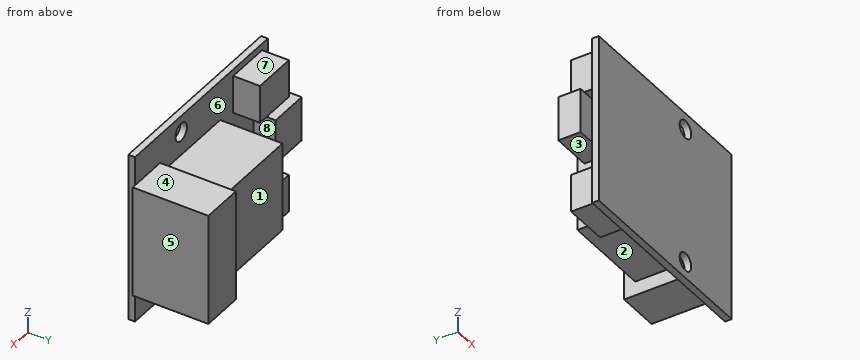
```python
from build123d import *

# Parameters (mm, degrees)
ESBO_O1_W                = 46
ESBO_O1_H                = 38
ESBO_O1_R                = 2
RESSALTO_EXTRUS_O1_DEPTH = 1.5
ESBO_O2_W                = 9
ESBO_O2_H                = 10
RESSALTO_EXTRUS_O2_DEPTH = 5
ESBO_O2_3_W              = 10
ESBO_O2_3_H              = 8.5
RESSALTO_EXTRUS_O3_DEPTH = 6
ESBO_O2_4_W              = 20
ESBO_O2_4_H              = 20
RESSALTO_EXTRUS_O4_DEPTH = 14
ESBO_O2_5_W              = 9.5
ESBO_O2_5_H              = 25
RESSALTO_EXTRUS_O5_DEPTH = 17


with BuildPart() as part:
    # Esboço1 → Ressalto-extrusão1 (new body)
    with BuildSketch(Plane(origin=(0, 0, 0), x_dir=(1, 0, 0), z_dir=(0, 1, 0))):
        Rectangle(ESBO_O1_W, ESBO_O1_H)
        with Locations((7, -15.3)):
            Circle(ESBO_O1_R, mode=Mode.SUBTRACT)
        with Locations((7, 15.3)):
            Circle(ESBO_O1_R, mode=Mode.SUBTRACT)
    extrude(amount=RESSALTO_EXTRUS_O1_DEPTH)

    # Esboço2 → Ressalto-extrusão2 (add)
    with BuildSketch(Plane(origin=(0, 1.5, 0), x_dir=(1, 0, 0), z_dir=(0, 1, 0))):
        with Locations((-22.5, 0)):
            Rectangle(ESBO_O2_W, ESBO_O2_H)
    extrude(amount=RESSALTO_EXTRUS_O2_DEPTH)

    # Esboço2<3> → Ressalto-extrusão3 (add)
    with BuildSketch(Plane(origin=(0, 1.5, 0), x_dir=(1, 0, 0), z_dir=(0, 1, 0))):
        with Locations((-16, -13.25)):
            Rectangle(ESBO_O2_3_W, ESBO_O2_3_H)
        with Locations((-16, 13.25)):
            Rectangle(ESBO_O2_3_W, ESBO_O2_3_H)
    extrude(amount=RESSALTO_EXTRUS_O3_DEPTH)

    # Esboço2<4> → Ressalto-extrusão4 (add)
    with BuildSketch(Plane(origin=(0, 1.5, 0), x_dir=(1, 0, 0), z_dir=(0, 1, 0))):
        with Locations((3.5, 0)):
            Rectangle(ESBO_O2_4_W, ESBO_O2_4_H)
    extrude(amount=RESSALTO_EXTRUS_O4_DEPTH)

    # Esboço2<5> → Ressalto-extrusão5 (add)
    with BuildSketch(Plane(origin=(0, 1.5, 0), x_dir=(1, 0, 0), z_dir=(0, 1, 0))):
        with Locations((19.05, 0)):
            Rectangle(ESBO_O2_5_W, ESBO_O2_5_H)
    extrude(amount=RESSALTO_EXTRUS_O5_DEPTH)


solid = part.part
```
Could you check a few things on this model? Use its own coordinates, in mm. Face numbers are marked on the shaded views. A direction names the side the tool comes from. Round coordinates to 2 decimals unless told otherwise and drop trailing zeros. Write each loop counter-clockwise with the first axis right and the second up, starting at its lowest first coordinate (ties: lowest second). Pieces come first, ordered by that corner, then holes. Notation, with made-up numbers: M -36,34 L -9,34 A5 ccw -9,41 Z; hole C 61.5,2.5 d9. An arc over 180 degrees is marked long. Write each question's results on one line, items separated by ' | '. Start each with the question number.
1. On a 3-axis mill with a long thin cutter (end or side, diameter ignored), from which of +Z, -Z, +X, -X, +Y, -Y can I reach the whole of each face in a straight line? I mean the marked faces 1, 2, 3 and 4. Say none if no direction works.
2. Thinking about a two-plate mould opening in X: for the marked faces 5, 6, 7 and 8, which applies, +X half, -X half, draft (parallel to the pull), parting line (faces both ways), or undercut?
3. Imagine slicing it at B-B on y = 2.5. List the corners of the cut face in (x, z) for me.
4. Imagine slicing it at C-C on x = 7. List the corners of the cut face in (y, z) for me.
5. I'm going to push flat-ended pins straight in: pin 1 Ø2 at (x, z) = (-24.5, 1.5) entering from -Y; pin 2 Ø1 at (x, y) = (18, 12) entering from +Z; pin 3 Ø1.8 at (x, y) = (-16, 4) entering from +Z. Where does each tip first touch, or does it pass through?
6. Imagine slicing it at D-D on y = 13.25. List the corners of the cut face in (x, z) for me, and give its area (4 significant figures).
7. Imagine slicing it at A-A on z = -15.3. List the corners of the cut face in (x, y) for me.
8. I need wall thicknesses on L1, parallel to Z at x = 7, y = 1.15; L2, parallel to X at y = 5, z = 0; L3, parallel to X at y = 2.5, z = 12. Which ranges of each line are inside material? Lowest first, please. Write a range as from..to.
Result sheet:
1) face 1: +Z, -Z, -X, +Y | face 2: -Z, +Y | face 3: -X, +Y | face 4: +Z, +X, +Y
2) face 5: +X half | face 6: undercut | face 7: draft | face 8: undercut
3) outline: M -27,-5 L -18,-5 L -18,5 L -27,5 Z; M -21,-17.5 L -11,-17.5 L -11,-9 L -21,-9 Z; M -21,9 L -11,9 L -11,17.5 L -21,17.5 Z; M -6.5,-10 L 13.5,-10 L 13.5,10 L -6.5,10 Z; M 14.3,-12.5 L 23.8,-12.5 L 23.8,12.5 L 14.3,12.5 Z
4) outline: M 0,-19 L 1.5,-19 L 1.5,-17.3 L 0,-17.3 Z; M 0,-13.3 L 1.5,-13.3 L 1.5,-10 L 15.5,-10 L 15.5,10 L 1.5,10 L 1.5,13.3 L 0,13.3 Z; M 0,17.3 L 1.5,17.3 L 1.5,19 L 0,19 Z
5) pin 1: stops at y = 1.5 | pin 2: stops at z = 12.5 | pin 3: stops at z = 17.5
6) outline: M -6.5,-10 L 13.5,-10 L 13.5,10 L -6.5,10 Z; M 14.3,-12.5 L 23.8,-12.5 L 23.8,12.5 L 14.3,12.5 Z | area: 637.5 mm^2
7) outline: M -23,0 L 5,0 L 5,1.5 L -11,1.5 L -11,7.5 L -21,7.5 L -21,1.5 L -23,1.5 Z; M 9,0 L 23,0 L 23,1.5 L 9,1.5 Z
8) L1: z = -19..-17.3, -13.3..13.3, 17.3..19 | L2: x = -27..-18, -6.5..13.5, 14.3..23.8 | L3: x = -21..-11, 14.3..23.8
